CAD build for the part. Positions are in the model's coordinates, mm. A direction names the side the tool comes from. Coordinates: 2 decimals unless noted, no trailing zeros. Write each loop counter-clockwise with the first axis right and the second up, starting at its lowest first coordinate (ties: lowest second). Pieces come first, ordered by that corner, then holes. Notation, with made-up numbers: M -21,-5 L 7,-5 A30 cw 7,18 Z; hole C 55.5,67 d1. An arc over 180 degrees is marked long. Answer as CSV lines item,"result". Start each with the question number.
```python
from build123d import *

# Parameters (mm, degrees)
ESQUISSE1_W        = 70
ESQUISSE1_H        = 30
ESQUISSE1_R        = 2.1
BOSS_EXTRU_1_DEPTH = 1.5


# Read off the part's stored shape, not the designer's step: PerçageAvancé1
with BuildPart() as part:
    # Esquisse1 → Boss.-Extru.1 (new, symmetric)
    with BuildSketch(Plane(origin=(0, 0, 0), x_dir=(1, 0, 0), z_dir=(0, 1, 0))):
        Rectangle(ESQUISSE1_W, ESQUISSE1_H)
        with Locations(Location((-20, 0, 0), (0, 0, 270))):
            Circle(ESQUISSE1_R, mode=Mode.SUBTRACT)
        with Locations(Location((20, 0, 0), (0, 0, 90))):
            Circle(ESQUISSE1_R, mode=Mode.SUBTRACT)
    extrude(amount=BOSS_EXTRU_1_DEPTH, both=True)

    # PerçageAvancé1 outline → PerçageAvancé1 (revolve, cut)
    with BuildSketch(Plane(origin=(-30, 0, 10), x_dir=(1, 0, 0), z_dir=(0, 0, 1))):
        Polygon((1.6, 0.05), (1.7, 0.05), (1.7, 1.5), (0, 1.5), (0, -1.5), (3.15, -1.5), align=None)
    revolve(axis=Axis((-30, 0, 10), (0, 1, 0)), mode=Mode.SUBTRACT)

    # Per_ageAvanc_1 2 outline → Per_ageAvanc_1 2 (revolve, cut)
    with BuildSketch(Plane(origin=(30, 0, 10), x_dir=(1, 0, 0), z_dir=(0, 0, 1))):
        Polygon((1.6, 0.05), (1.7, 0.05), (1.7, 1.5), (0, 1.5), (0, -1.5), (3.15, -1.5), align=None)
    revolve(axis=Axis((30, 0, 10), (0, 1, 0)), mode=Mode.SUBTRACT)

    # Per_ageAvanc_1 3 outline → Per_ageAvanc_1 3 (revolve, cut)
    with BuildSketch(Plane(origin=(30, 0, -10), x_dir=(1, 0, 0), z_dir=(0, 0, 1))):
        Polygon((1.6, 0.05), (1.7, 0.05), (1.7, 1.5), (0, 1.5), (0, -1.5), (3.15, -1.5), align=None)
    revolve(axis=Axis((30, 0, -10), (0, 1, 0)), mode=Mode.SUBTRACT)

    # Per_ageAvanc_1 4 outline → Per_ageAvanc_1 4 (revolve, cut)
    with BuildSketch(Plane(origin=(-30, 0, -10), x_dir=(1, 0, 0), z_dir=(0, 0, 1))):
        Polygon((1.6, 0.05), (1.7, 0.05), (1.7, 1.5), (0, 1.5), (0, -1.5), (3.15, -1.5), align=None)
    revolve(axis=Axis((-30, 0, -10), (0, 1, 0)), mode=Mode.SUBTRACT)


solid = part.part
```
1) Band-saw the part on B-B, the plane z = -10. List the corners of the cut face in (x, y), plus the area to 3 significant figures.
2) Tool access for faces 5 (the flat face through (0, 0, 15)), 6 (the cylindrical face through (31.57, 0.79, -9.35)): list every direction of +Z, -Z, +X, -X, +Y, -Y with a clear straight run to the whole face (end or side of a thin tool).
3) Band-saw the part on D-D, the plane x = 30. List the corners of the cut face in (y, z).
4) Band-saw the part on C-C, the plane y = 0.6. List the corners of the cut face in (x, z), plus the area to 3 significant figures.
5) Pin check, flat tip, straight feed: P1, Ø4, axis at x = 30, z = -10, coming from the -Y side. Stop position of the tip, or through.
6) Probe L1, parallel to X at y = 1.2, z = -10; L2, parallel to X at y = 0.65, z = 0; L3, parallel to Z at x = 30, y = 1.2. List the from-to ranges inside material, lowest first. Write a range as [from, to].
7) Band-saw the part on A-A, the plane x = 20. List the corners of the cut face in (y, z).
8) Two-plate mould, pull along X, no slides. Class faces 1 (the flat face through (-35, 0, 0)), 2 (the flat face through (0, 1.5, 0)), 3 (the cylindrical face through (-28.43, 0.79, 10.65)), 4 (the flat face through (35, 0, 0)): pulls with the +X half, pulls with the -X half, needs draft (parallel to the pull), parting line crosses it, or undercut.
Result sheet:
1,outline,"M -35,-1.5 L -33.15,-1.5 L -31.6,0.05 L -31.7,0.05 L -31.7,1.5 L -35,1.5 Z; M -28.4,0.05 L -26.85,-1.5 L 26.85,-1.5 L 28.4,0.05 L 28.3,0.05 L 28.3,1.5 L -28.3,1.5 L -28.3,0.05 Z; M 31.6,0.05 L 33.15,-1.5 L 35,-1.5 L 35,1.5 L 31.7,1.5 L 31.7,0.05 Z"
1,area,"185 mm²"
2,face 5,"+Z, +X, -X, +Y, -Y"
2,face 6,"+Y"
3,outline,"M -1.5,-15 L 1.5,-15 L 1.5,-11.7 L 0.05,-11.7 L 0.05,-11.6 L -1.5,-13.15 Z; M -1.5,-6.85 L 0.05,-8.4 L 0.05,-8.3 L 1.5,-8.3 L 1.5,8.3 L 0.05,8.3 L 0.05,8.4 L -1.5,6.85 Z; M -1.5,13.15 L 0.05,11.6 L 0.05,11.7 L 1.5,11.7 L 1.5,15 L -1.5,15 Z"
4,outline,"M -35,-15 L 35,-15 L 35,15 L -35,15 Z; hole C -30,-10 d3.4; hole C -30,10 d3.4; hole C -20,0 d4.2; hole C 20,0 d4.2; hole C 30,-10 d3.4; hole C 30,10 d3.4"
4,area,"2,040 mm²"
5,P1,"stops at y = -0.35"
6,L1,"x = [-35, -31.7], [-28.3, 28.3], [31.7, 35]"
6,L2,"x = [-35, -22.1], [-17.9, 17.9], [22.1, 35]"
6,L3,"z = [-15, -11.7], [-8.3, 8.3], [11.7, 15]"
7,outline,"M -1.5,-15 L 1.5,-15 L 1.5,-2.1 L -1.5,-2.1 Z; M -1.5,2.1 L 1.5,2.1 L 1.5,15 L -1.5,15 Z"
8,face 1,"pulls with the -X half"
8,face 2,"needs draft"
8,face 3,"undercut"
8,face 4,"pulls with the +X half"
